Part print with two shaded views. Sizes in mm from the minimum x, y, z corner. A direction names the side the tool comes from. Give positions to 0.01 mm unless a question says otherwise; leave off trailing zeros. Loops run counter-clockwise (first coordinate to the right, second up) from the corner with the lowest first, then second, coordinate; pieces in that order, holes last. Notation, with made-up numbers: M -34,56.25 L -17,56.25 A28 ccw -17,89.25 Z; hole C 68,89.5 d10. An arc over 180 degrees is marked long. Answer as a JSON object with one key per item and string values. Group by question number.
1. Mould opens along Y. For the marked faces 5, 6 and 7 say: released by +Y, released by -Y, zero draft, split by the parting line, or undercut.
2. Drill centre lines: line 1 along X through (y, z) = (18, 47) (1 decimal); line 2 along X through (y, z) = (37.5, 10) (1 decimal); line 3 along Z through (x, y) = (100, 56). Where is each one in solid material? Low to high. Write a range as [from, to].
3. Drop flat-ended pins along their axis: pin 1 Ø3 at (x, z) = (40.5, 45) entering from -Y; pin 2 Ø4 at (x, z) = (88.5, 8) entering from -Y; pin 3 Ø8 at (x, y) = (22, 33) entering from +Z. Give the stop position or say it passes through.
4. Slice it at A-A (z = 45). Give the number of separate pieces and of enclosed holes in the cut face, then the cut area to 3 significant figures.
5. 3-axis set-ups, long thin cutter, end or side, ignore diameter. For the marked faces 1, 2, 3 and 4: which of +Z, -Z, +X, -X, +Y, -Y reach the whole face in a straight line?
6. Slice it at B-B (x = 13). List the corners of the cut face in (y, z).
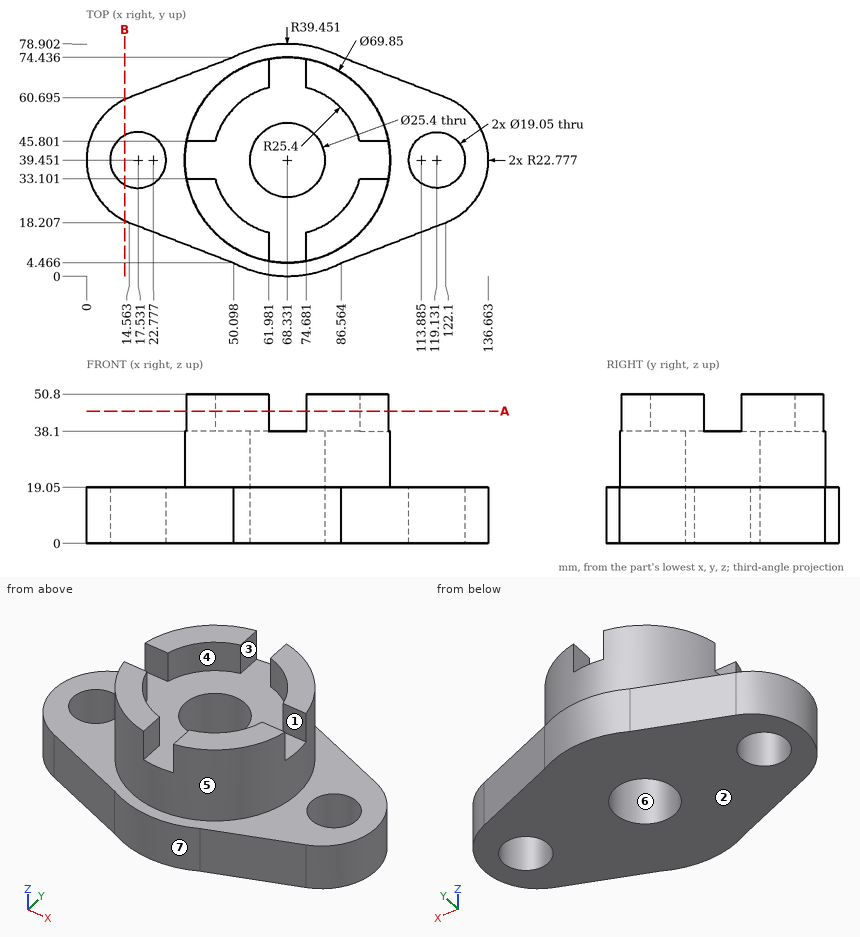
Established:
{
 "1": {"face 5": "split by the parting line", "face 6": "undercut", "face 7": "released by -Y"},
 "2": {"line 1": "x = [40.8, 54.7], [81.9, 95.9]", "line 2": "x = [0.1, 8.2], [26.9, 55.8], [80.9, 109.8], [128.5, 136.6]", "line 3": "z = [0, 19.05]"},
 "3": {"pin 1": "stops at y = 16.51", "pin 2": "stops at y = 4.43", "pin 3": "stops at z = 19.05"},
 "4": {"separate pieces": "4", "enclosed holes": "0", "area": "1,320 mm^2"},
 "5": {"face 1": "+Z, +X, -X", "face 2": "-Z, +X, -X, +Y, -Y", "face 3": "+Z, +Y, -Y", "face 4": "+Z"},
 "6": {"outline": "M 18.88,0 L 31.07,0 L 31.07,19.05 L 18.88,19.05 Z; M 47.83,0 L 60.02,0 L 60.02,19.05 L 47.83,19.05 Z"}
}
